Build history of the part. All positions in model axes, mm. Give positions to 0.01 mm unless a question says otherwise; leave off trailing zeros. Order: outer loops, then holes, each group sorted by start corner. A loop starts at its lowest first (then second) coordinate and runs counter-clockwise, first axis right, second up. Notation, with made-up numbers: (-17, 33) - (-11, 33) arc R15 ccw to (-11, 47) - close; hole circle Ø1 at (73, 7.25). An arc over 180 degrees is marked (long way). Use a Markdown table: item, result. Add a question column.
(1) Flat gauge pins, fed straight in: pin 1 (3.5 mm diameter, centred on x = 0, y = 25, fed in from -Z); pin 2 (1.5 mm diameter, centred on y = 21, z = 1.5, fed in from +X); pin 3 (2 mm diameter, centred on x = 8.5, z = 1.5, fed in from +Y); pin 4 (1 mm diameter, centred on x = -23.5, y = 17, fed in from +Z). Where does each tip first touch, or does it go through?
(2) Wall check: line 1 (Y direction, x = 0, z = 0.6); line 2 (Y direction, x = 23, z = 4.35); line 3 (Y direction, x = -22.5, z = 2.75). Give the ranges that are in metal, low to high.
(3) Slice it at C-C (z = 4.15). Write the cut outline in (x, y), then the cut area to 3 significant figures.
(4) Mould opens along Y. For faces 1 (the face through (13, 0, 0)), 2 (the face through (-2.38, -10.74, 1.48)), 3 (the face through (23.7, -13.3, 2.5)), 4 (the face through (-29.97, 1.32, 1.48)) say: +Y half, -Y half, draft (parallel to the pull), parting line (faces both ways), or undercut.
(5) Slice it at B-B (y = 0). Write the cut outline in (x, z).
(6) Slice it at A-A (x = 0). Write the cut outline in (y, z), then the cut area to 3 significant figures.
from build123d import *

# Parameters (mm, degrees)
F0_R     = 30
F0_R_2   = 2.2
F0_R_3   = 11
F1_DEPTH = 5
F2_R     = 2
F3_R     = 2


with BuildPart() as f1:
    # F0 (on Top) → F1 (new body)
    with BuildSketch(Plane.XY):
        Circle(F0_R)
        with Locations((-21.650635, -12.5)):
            Circle(F0_R_2, mode=Mode.SUBTRACT)
        with Locations((0, -25)):
            Circle(F0_R_2, mode=Mode.SUBTRACT)
        with Locations((21.650635, -12.5)):
            Circle(F0_R_2, mode=Mode.SUBTRACT)
        with Locations((-21.650635, 12.5)):
            Circle(F0_R_2, mode=Mode.SUBTRACT)
        Circle(F0_R_3, mode=Mode.SUBTRACT)
        with Locations((21.650635, 12.5)):
            Circle(F0_R_2, mode=Mode.SUBTRACT)
        with Locations((0, 25)):
            Circle(F0_R_2, mode=Mode.SUBTRACT)
    extrude(amount=F1_DEPTH)

    # F2
    f2_edges = [f1.edges().sort_by_distance(p)[0] for p in [
        (-30, 0, 5),
    ]]
    fillet(f2_edges, radius=F2_R)

    # F3
    f3_edges = [f1.edges().sort_by_distance(p)[0] for p in [
        (-11, 0, 5),
    ]]
    fillet(f3_edges, radius=F3_R)


solid = f1.part
Solution:
| question | item | result |
|---|---|---|
| 1 | pin 1 | through |
| 1 | pin 2 | x = 22.13 |
| 1 | pin 3 | y = 29.05 |
| 1 | pin 4 | z = 4.94 |
| 2 | line 1 | -30 to -27.2, -22.8 to -11, 11 to 22.8, 27.2 to 30 |
| 2 | line 2 | -18.43 to -14.24, -10.76 to 10.76, 14.24 to 18.43 |
| 2 | line 3 | -19.84 to -14.53, -10.47 to 10.47, 14.53 to 19.84 |
| 3 | outline | circle Ø59.27 at (0, 0); hole circle Ø4.4 at (-21.65, -12.5); hole circle Ø4.4 at (-21.65, 12.5); hole circle Ø22.73 at (0, 0); hole circle Ø4.4 at (0, -25); hole circle Ø4.4 at (0, 25); hole circle Ø4.4 at (21.65, -12.5); hole circle Ø4.4 at (21.65, 12.5) |
| 3 | area | 2,260 mm2 |
| 4 | face 1 | draft |
| 4 | face 2 | undercut |
| 4 | face 3 | undercut |
| 4 | face 4 | parting line |
| 5 | outline | (-30, 0) - (-11, 0) - (-11, 3) arc R2 ccw to (-13, 5) - (-28, 5) arc R2 ccw to (-30, 3) - close; (11, 0) - (30, 0) - (30, 3) arc R2 ccw to (28, 5) - (13, 5) arc R2 ccw to (11, 3) - close |
| 6 | outline | (-30, 0) - (-27.2, 0) - (-27.2, 5) - (-28, 5) arc R2 ccw to (-30, 3) - close; (-22.8, 0) - (-11, 0) - (-11, 3) arc R2 ccw to (-13, 5) - (-22.8, 5) - close; (11, 0) - (22.8, 0) - (22.8, 5) - (13, 5) arc R2 ccw to (11, 3) - close; (27.2, 0) - (30, 0) - (30, 3) arc R2 ccw to (28, 5) - (27.2, 5) - close |
| 6 | area | 143 mm2 |
